Autodesk Inventor part; units mm, degrees
ref_plane "YZ Plane" through (0, 0, 0) normal (1, 0, 0) x (0, 1, 0)
ref_plane "XZ Plane" through (0, 0, 0) normal (0, 1, 0) x (-1, 0, 0)
ref_plane "XY Plane" through (0, 0, 0) normal (0, 0, 1) x (1, 0, 0)
sketch "Sketch1" plane through (0, 0, 0) normal (0, 1, 0) x (-1, 0, 0)
  line L0 (-8.001, 0) -> (8.001, 0) construction
  line L1 (-8.001, -4.191) -> (8.001, -4.191)
  line L2 (8.001, 4.191) -> (-8.001, 4.191)
  arc A0 (-8.001, 4.191) -> (-8.001, -4.191) centre (-8.001, 0) ccw
  arc A1 (8.001, -4.191) -> (8.001, 4.191) centre (8.001, 0) ccw
  line L3 (-2.6941, 0) -> (0, 2.6941)
  line L4 (0, 2.6941) -> (2.6941, 0)
  line L5 (2.6941, 0) -> (0, -2.6941)
  line L6 (0, -2.6941) -> (-2.6941, 0)
  line L7 (-2.6941, 0) -> (2.6941, 0) construction
  line L8 (0, 2.6941) -> (0, -2.6941) construction
  point P0 (0, 0)
  dimension "d0" = 8.001
  dimension "d1" = 8.382
  dimension "d2" = 3.81
  dimension "d3" = 3.81
extrude "Extrusion1" add sketch "Sketch1" along normal blind 7.493
sketch "Sketch2" plane through (0, 7.493, 0) normal (0, 1, 0) x (1, 0, 0)
  circle A0 centre (-8.001, 0) radius 3.2385
  point P0 (0, 0)
  dimension "d6" = 8.001
  dimension "d7" = 6.477
extrude "Extrusion2" cut sketch "Sketch2" against normal blind 0.7874
sketch "Sketch3" plane through (0, 7.493, 0) normal (0, 1, 0) x (1, 0, 0)
  circle A0 centre (8.001, 0) radius 3.2385
  point P0 (0, 0)
  dimension "d10" = 8.001
  dimension "d11" = 6.477
extrude "Extrusion3" cut sketch "Sketch3" against normal blind 0.7874
sketch "Sketch4" plane through (0, 0, 0) normal (0, -1, 0) x (1, 0, 0)
  circle A0 centre (8.001, 0) radius 3.2385
  circle A1 centre (8.001, 0) radius 2.8575
  point P0 (0, 0)
extrude "Extrusion4" cut sketch "Sketch4" against normal blind 0.7874 contours A0 | A1
sketch "Sketch5" plane through (0, 0, 0) normal (0, -1, 0) x (1, 0, 0)
  circle A0 centre (-8.001, 0) radius 3.2385
  circle A1 centre (-8.001, 0) radius 2.8575
  point P0 (0, 0)
extrude "Extrusion5" cut sketch "Sketch5" against normal blind 0.7874 contours A0 | A1
sketch "Sketch6" plane through (-8.001, 6.7056, 0) normal (0, 1, 0) x (1, 0, 0)
  circle A0 centre (0, 0) radius 2.7051
  point P0 (8.001, 0)
  dimension "d18" = 5.4102
extrude "Extrusion6" cut sketch "Sketch6" against normal through all
sketch "Sketch7" plane through (8.001, 6.7056, 0) normal (0, 1, 0) x (1, 0, 0)
  circle A0 centre (0, 0) radius 2.7051
  point P0 (-8.001, 0)
  dimension "d21" = 5.4102
extrude "Extrusion7" cut sketch "Sketch7" against normal through all
properties part number "VexLegoBiggerCoupler"
Read the model definition and answer for the solid it produces. Units are mm, in the model's axes. A direction names the side the tool comes from. Coordinates: 2 decimals unless noted, no trailing zeros. Write each loop counter-clockwise with the first axis right and the second up, starting at its lowest first coordinate (ties: lowest second). Pieces come first, ordered by that corner, then holes. Notation, with made-up numbers: (-16, 5.5) -> (29, 5.5) arc R19 ccw to (29, 25.5) -> close; hole circle Ø3 at (3, 67.25). An arc over 180 degrees is marked (long way). Return JSON: item names as keys, results as strings.
1. A cutting plane is placed at B-B (x = 5.75). Determine the outline of the cut face in (y, z), and give its area (3 significant figures).
Found:
{"outline": "(0, -4.19) -> (7.49, -4.19) -> (7.49, -2.33) -> (6.71, -2.33) -> (6.71, -1.5) -> (0.79, -1.5) -> (0.79, -2.33) -> (0, -2.33) -> close; (0, 2.33) -> (0.79, 2.33) -> (0.79, 1.5) -> (6.71, 1.5) -> (6.71, 2.33) -> (7.49, 2.33) -> (7.49, 4.19) -> (0, 4.19) -> close", "area": "37.7 mm2"}
2. A cutting plane is placed at C-C (z = -1.5). Give the number of separate pieces and of enclosed holes in the cut face, and give its area (3 significant figures).
Found:
{"separate pieces": "4", "enclosed holes": "0", "area": "89.3 mm2"}
3. Determine the mould class of faces 5 (the face through (-5.42, 3.79, -0.81)), 6 (the face through (3, 0, 0)), 7 (the face through (0, 4, -4.191)) for opening direction Z: pulls with the +Z half, pulls with the -Z half, needs draft (parallel to the pull), parting line crosses it, or undercut.
Found:
{"face 5": "undercut", "face 6": "needs draft", "face 7": "pulls with the -Z half"}
4. Find the intervals of material crossed by line 1 along X through (y, z) = (6.75, 1.25); line 2 along X through (y, z) = (7.25, -2.25); line 3 along Y through (x, z) = (5.5, 2), in increasing order. Write a range as from..to.
Found:
{"line 1": "-12..-10.99, -5.01..-1.44, 1.44..5.01, 10.99..12", "line 2": "-11.54..-10.33, -5.67..-0.44, 0.44..5.67, 10.33..11.54", "line 3": "0.79..6.71"}
5. A tool of negligible diameter and unlimited length cuts with its end or side. For faces 1 (the face through (4.766, 7.105, -0.142)), 2 (the face through (-12.19, 3.69, 0.09)), 3 (the face through (-5.01, 0.39, -1.24)), 4 (the face through (1.366, 3.694, 1.328)), from which of +Z, -Z, +X, -X, +Y, -Y can it reach the whole face along a straight path? Write none if from no direction.
Found:
{"face 1": "+Y", "face 2": "-X, +Y, -Y", "face 3": "-Y", "face 4": "+Y, -Y"}
6. A cutting plane is placed at A-A (y = 3.75). Determine the outline of the cut face in (x, z), and give its area (3 significant figures).
Found:
{"outline": "(-8, -4.19) -> (8, -4.19) arc R4.19 ccw to (8, 4.19) -> (-8, 4.19) arc R4.19 ccw to start; hole circle Ø5.41 at (-8, 0); hole (-2.69, 0) -> (0, -2.69) -> (2.69, 0) -> (0, 2.69) -> close; hole circle Ø5.41 at (8, 0)", "area": "129 mm2"}
7. Each of these flat-tipped pins is pushed along its axis until it touches: P1, Ø1, axis at y = 5.5, z = 2.5, coming from the -X side; P2, Ø1.5, axis at y = 5, z = -1.5, coming from the -X side; P3, Ø1.5, axis at y = 4.5, z = 2, coming from the -X side. Where does it stop, or does it pass through?
Found:
{"P1": "x = -11.68", "P2": "x = -12.12", "P3": "x = -12"}
8. A cutting plane is placed at D-D (x = -9.5). Determine the outline of the cut face in (y, z).
Found:
{"outline": "(0, -3.91) -> (7.49, -3.91) -> (7.49, -2.87) -> (6.71, -2.87) -> (6.71, -2.25) -> (0.79, -2.25) -> (0.79, -2.87) -> (0, -2.87) -> close; (0, 2.87) -> (0.79, 2.87) -> (0.79, 2.25) -> (6.71, 2.25) -> (6.71, 2.87) -> (7.49, 2.87) -> (7.49, 3.91) -> (0, 3.91) -> close"}
